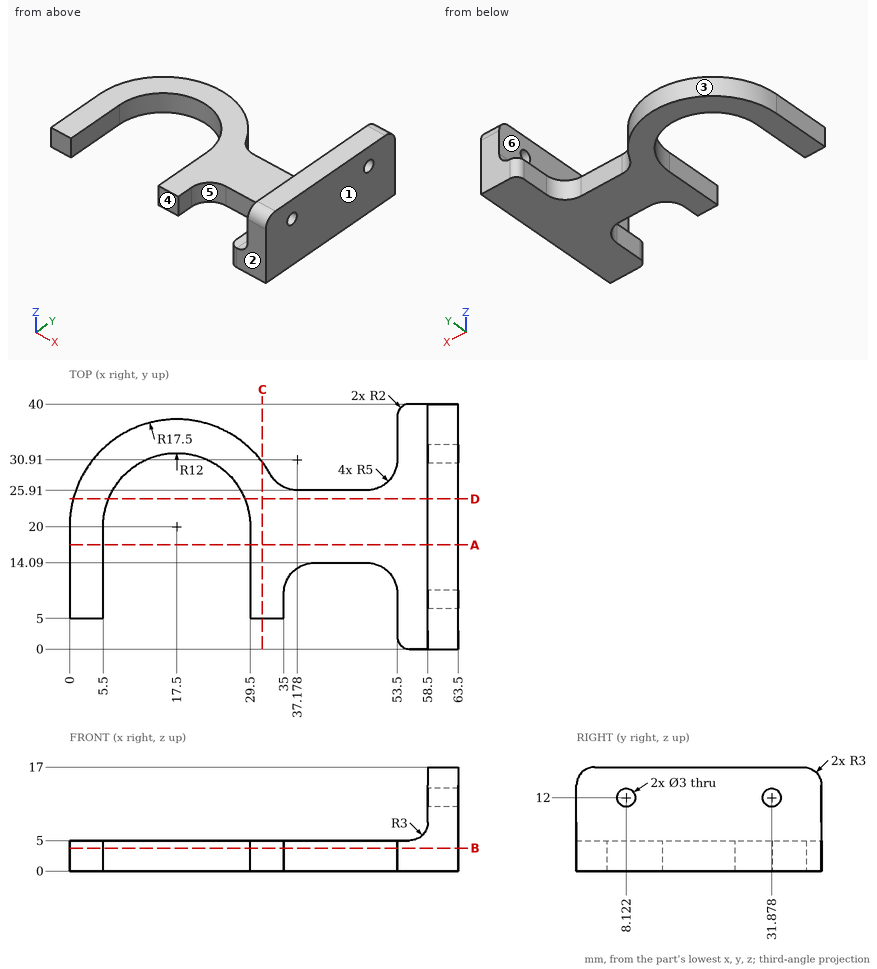
Study the drawing (mm; zero at the part's minimum x, y, z) and answer. A direction names the side the tool comes from. Give positions to 0.01 mm unless a question says otherwise; leave off trailing zeros. Order: outer loops, then holes, each group sorted by start corner. A loop starts at its lowest first (then second) coordinate and runs counter-clockwise, first axis right, second up. Notation, with made-up numbers: (48.25, 2) -> (83.25, 2) arc R24 cw to (83.25, 12) -> close; hole circle Ø5 at (81, 42). An arc over 180 degrees is marked (long way). Put each result on its own line as item: value.
Item 1: Straight lines are drawn through the part: line 1 (X direction, y = 4, z = 3.75); line 2 (X direction, y = 34, z = 10.25); line 3 (X direction, y = 31, z = 4.75) (1 decimal). For each, find the intervals that lie inside material, in ascending order.
Established:
line 1: x = 53.5 to 63.5
line 2: x = 58.5 to 63.5
line 3: x = 3.9 to 12.7, 22.3 to 31.1, 53.5 to 63.5
Item 2: A cutting plane is placed at A-A on y = 17. Give the vertices of the cut face in (x, z).
Established:
outline: (0, 0) -> (5.5, 0) -> (5.5, 5) -> (0, 5) -> close; (29.5, 0) -> (63.5, 0) -> (63.5, 17) -> (58.5, 17) -> (58.5, 8) arc R3 cw to (55.5, 5) -> (29.5, 5) -> close
Item 3: A cutting plane is placed at C-C on x = 31.5. Give the vertices of the cut face in (y, z).
Established:
outline: (5, 0) -> (30.5, 0) -> (30.5, 5) -> (5, 5) -> close
Item 4: Given P1, Ø6, axis at y = 27, z = 4, coming from the -X side; P2, Ø1.5, axis at x = 3, z = 3, coming from the -Y side; P3, Ø20, axis at x = 37, y = 17.5, coming from the +Z side, each flat-ended and moving along its own axis, determine where each tip first touches the part or whether it passes through.
Established:
P1: stops at x = 0.46
P2: stops at y = 5
P3: stops at z = 5
Item 5: For the marked faces 4, 5 and 6, determine the directions among +Z, -Z, +X, -X, +Y, -Y from which every point of the face is accessible in a straight line to the end or side of a thin tool.
Established:
face 4: +Z, -Z, -X, -Y
face 5: +Z, -Z, -Y
face 6: +Z, -X, +Y, -Y
Item 6: A cutting plane is placed at B-B on z = 3.75. Give the vertices of the cut face in (x, y) (1 decimal).
Established:
outline: (0, 5) -> (5.5, 5) -> (5.5, 20) arc R12 cw to (29.5, 20) -> (29.5, 5) -> (35, 5) -> (35, 9.1) arc R5 cw to (40, 14.1) -> (48.5, 14.1) arc R5 cw to (53.5, 9.1) -> (53.5, 2) arc R2 ccw to (55.5, 0) -> (63.5, 0) -> (63.5, 40) -> (55.5, 40) arc R2 ccw to (53.5, 38) -> (53.5, 30.9) arc R5 cw to (48.5, 25.9) -> (37.2, 25.9) arc R5 cw to (32.8, 28.5) arc R17.5 ccw to (0, 20) -> close
Item 7: A cutting plane is placed at D-D on y = 24.5. Give the vertices of the cut face in (x, z) (1 decimal), plus the area to 3 significant figures.
Established:
outline: (0.6, 0) -> (6.4, 0) -> (6.4, 5) -> (0.6, 5) -> close; (28.6, 0) -> (63.5, 0) -> (63.5, 17) -> (58.5, 17) -> (58.5, 8) arc R3 cw to (55.5, 5) -> (28.6, 5) -> close
area: 265 mm^2
Item 8: For a pull along X with two mould halves and no side action, classify the marked faces 1, 2 and 3 as released by +X, released by -X, zero draft, split by the parting line, or undercut.
Established:
face 1: released by +X
face 2: zero draft
face 3: undercut
